Design review of the part built by this model. Coordinates are the model's own, in mm. Coordinates: 2 decimals unless noted, no trailing zeros. Loops run counter-clockwise (first coordinate to the right, second up) from the corner with the lowest first, then second, coordinate; pieces in that order, holes last. Notation, with made-up numbers: M 70,24 L 79,24 A31 cw 79,60 Z; hole C 51,8.5 d6. An arc over 180 degrees is marked long. Put each result on its own line as item: value. Start each with the question number.
(1) Take a section at C-C, the plane x = 5.5. Give the boundary of the cut face in (y, z).
(2) Take a section at D-D, the plane z = 4.5. Give the boundary of the cut face in (x, y).
(3) The part is to be moulded in two halves that separate along Y. For faces 1 (the flat face through (-21, 39, 5.715)), 2 (the cylindrical face through (36.651, 0.889, 4.822)), 3 (the cylindrical face through (-0.533, 62.051, 4.822)), say which applies: +Y half, -Y half, draft (parallel to the pull), parting line (faces both ways), or undercut.
(4) For probe 1 along Z at (x, y) = (31.5, -27.5); probe 2 along X at (y, z) = (24, 1.5); probe 3 along X at (y, z) = (-52, 3.75), list the stretches that pass through material, from the lowest coordinate up. Write a range as [from, to].
(5) Take a section at A-A, the plane x = -20.5. Give the boundary of the cut face in (y, z) (3 decimals).
(6) Clearance check with flat-ended pins moving along their axes: pin 1 (2 mm diameter, centred on x = 12, z = 5.5, fed in from -Y); pin 2 (1 mm diameter, centred on x = 5.5, y = 47, fed in from +Z); pin 3 (3 mm diameter, centred on x = -19, z = 4, fed in from +Y). State where each tip first meets the part, or that it passes through.
(7) Take a section at B-B, the plane y = -40. Give the boundary of the cut face in (x, z).
```python
from build123d import *

# Parameters (mm, degrees)
F0_W        = 76.2
F0_H        = 127
F1_DEPTH    = 6.35
F2_W        = 12.7
F2_H        = 12.7
F3_DEPTH    = 1.27
F4_W        = 6.35
F4_H        = 6.35
F5_DEPTH    = 0.635
F6_T1_DEPTH = 29.5005208253
F6_T3_DEPTH = 29.5005208253
F6_T5_DEPTH = 152.4
F6_T7_DEPTH = 101.6


# Not quite as in the source:
# - a fillet or chamfer that OpenCascade refuses, or shapes differently, is made with other operations: its cross-section is extruded or revolved along the edge and cut away or added


with BuildPart() as f1:
    # F0 (on Top) → F1 (new body)
    with BuildSketch(Plane.XY):
        Rectangle(F0_W, F0_H)
    extrude(amount=F1_DEPTH)

    # F2 (on face) → F3 (join)
    with BuildSketch(Plane.XY.offset(6.35)):
        with Locations((3.8891917182, 42.4066188663)):
            Rectangle(F2_W, F2_H)
    extrude(amount=F3_DEPTH)

    # F4 (on face) → F5 (cut)
    with BuildSketch(Plane.XY.offset(6.35)):
        with Locations((-20.5224687852, 39.1501502216)):
            Rectangle(F4_W, F4_H)
    extrude(amount=-F5_DEPTH, mode=Mode.SUBTRACT)

    # F6: fillet of radius 5.08 on 8 edges, made by hand

    # F6_s2 → F6_t1 (cut)
    with BuildSketch(Plane.XZ.offset(-57.156879279)):
        with BuildLine():
            ThreePointArc((10.2391917182, 6.35), (8.6751387773, 7.2919048812), (6.8790875531, 7.62))
            Line((6.8790875531, 7.62), (10.2391917182, 7.62))
            Line((10.2391917182, 7.62), (10.2391917182, 6.35))
        make_face()
        with BuildLine():
            ThreePointArc((-2.4608082818, 6.35), (-0.896755341, 7.2919048812), (0.8992958832, 7.62))
            Line((0.8992958832, 7.62), (-2.4608082818, 7.62))
            Line((-2.4608082818, 7.62), (-2.4608082818, 6.35))
        make_face()
    extrude(amount=F6_T1_DEPTH, mode=Mode.SUBTRACT)

    # F6_s4 → F6_t3 (cut)
    with BuildSketch(Plane.YZ.offset(-10.8610686945)):
        with BuildLine():
            ThreePointArc((48.7566188663, 6.35), (47.1925659255, 7.2919048812), (45.3965147013, 7.62))
            Line((45.3965147013, 7.62), (48.7566188663, 7.62))
            Line((48.7566188663, 7.62), (48.7566188663, 6.35))
        make_face()
        with BuildLine():
            ThreePointArc((36.0566188663, 6.35), (37.6206718072, 7.2919048812), (39.4167230314, 7.62))
            Line((39.4167230314, 7.62), (36.0566188663, 7.62))
            Line((36.0566188663, 7.62), (36.0566188663, 6.35))
        make_face()
    extrude(amount=F6_T3_DEPTH, mode=Mode.SUBTRACT)

    # F6_s6 → F6_t5 (cut)
    with BuildSketch(Plane.XZ.offset(-76.2)):
        with BuildLine():
            ThreePointArc((38.1, 1.27), (36.6121024484, 4.8621024484), (33.02, 6.35))
            Line((33.02, 6.35), (38.1, 6.35))
            Line((38.1, 6.35), (38.1, 1.27))
        make_face()
        with BuildLine():
            ThreePointArc((-33.02, 6.35), (-36.6121024484, 4.8621024484), (-38.1, 1.27))
            Line((-38.1, 1.27), (-38.1, 6.35))
            Line((-38.1, 6.35), (-33.02, 6.35))
        make_face()
    extrude(amount=F6_T5_DEPTH, mode=Mode.SUBTRACT)

    # F6_s8 → F6_t7 (cut)
    with BuildSketch(Plane.YZ.offset(-50.8)):
        with BuildLine():
            ThreePointArc((-63.5, 1.27), (-62.0121024484, 4.8621024484), (-58.42, 6.35))
            Line((-58.42, 6.35), (-63.5, 6.35))
            Line((-63.5, 6.35), (-63.5, 1.27))
        make_face()
        with BuildLine():
            ThreePointArc((63.5, 1.27), (62.0121024484, 4.8621024484), (58.42, 6.35))
            Line((58.42, 6.35), (63.5, 6.35))
            Line((63.5, 6.35), (63.5, 1.27))
        make_face()
    extrude(amount=F6_T7_DEPTH, mode=Mode.SUBTRACT)


solid = f1.part
```
Computed values:
1. outline: M -63.5,0 L 63.5,0 L 63.5,1.27 A5.08 ccw 58.42,6.35 L 48.76,6.35 A5.08 ccw 45.4,7.62 L 39.42,7.62 A5.08 ccw 36.06,6.35 L -58.42,6.35 A5.08 ccw -63.5,1.27 Z
2. outline: M -36.94,-62.34 L 36.94,-62.34 L 36.94,62.34 L -36.94,62.34 Z
3. face 1: undercut
3. face 2: draft
3. face 3: +Y half
4. probe 1: z = [0, 6.35]
4. probe 2: x = [-38.09, 38.09]
4. probe 3: x = [-37.45, 37.45]
5. outline: M -63.5,0 L 63.5,0 L 63.5,1.27 A5.08 ccw 58.42,6.35 L 42.325,6.35 L 42.325,5.715 L 35.975,5.715 L 35.975,6.35 L -58.42,6.35 A5.08 ccw -63.5,1.27 Z
6. pin 1: stops at y = -62.34
6. pin 2: stops at z = 7.5
6. pin 3: stops at y = 63.35
7. outline: M -38.1,0 L 38.1,0 L 38.1,1.27 A5.08 ccw 33.02,6.35 L -33.02,6.35 A5.08 ccw -38.1,1.27 Z
